Read the model definition and answer for the solid it produces. Units are mm, in the model's axes. Face numbers are marked on the shaded views. A direction names the side the tool comes from. Coordinates: 2 decimals unless noted, no trailing zeros. Order: outer loops, then holes, each group sorted by start corner. A loop starts at its lowest first (then second) coordinate and runs counter-clockwise, first axis right, second up.
```python
from build123d import *

# Parameters (mm, degrees)
SKETCH1_R           = 17
BOSS_EXTRUDE1_DEPTH = 14
SKETCH2_R           = 12.9
CUT_EXTRUDE1_DEPTH  = 10.5
SKETCH3_R           = 11
CUT_EXTRUDE3_DEPTH  = 28.820855486


with BuildPart() as part:
    # Sketch1 → Boss-Extrude1 (new body)
    with BuildSketch(Plane.XY):
        Circle(SKETCH1_R)
    extrude(amount=BOSS_EXTRUDE1_DEPTH)

    # Sketch2 → Cut-Extrude1 (cut)
    with BuildSketch(Plane.XY):
        with Locations(Location((0, 0, 0), (0, 0, 180))):
            Circle(SKETCH2_R)
    extrude(amount=CUT_EXTRUDE1_DEPTH, mode=Mode.SUBTRACT)

    # Sketch3 → Cut-Extrude3 (cut, through all)
    with BuildSketch(Plane.XY):
        Circle(SKETCH3_R)
    extrude(amount=CUT_EXTRUDE3_DEPTH, mode=Mode.SUBTRACT)


solid = part.part
```
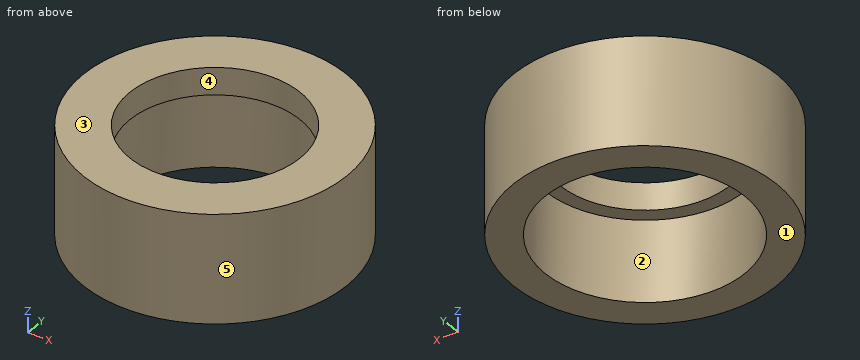
1) Straight lines are drawn through the part: line 1 (Y direction, x = 0, z = 5); line 2 (Y direction, x = 0, z = 11.4); line 3 (Z direction, x = -10.5, y = 6.5). For each, find the intervals that lie inside material, in ascending order.
A:
line 1: y = -17 to -12.9, 12.9 to 17
line 2: y = -17 to -11, 11 to 17
line 3: z = 10.5 to 14
2) A cutting plane is placed at B-B, the plane x = -4. Determine the outline of the cut face in (y, z).
A:
outline: (-16.52, 0) - (-12.26, 0) - (-12.26, 10.5) - (-10.25, 10.5) - (-10.25, 14) - (-16.52, 14) - close; (10.25, 10.5) - (12.26, 10.5) - (12.26, 0) - (16.52, 0) - (16.52, 14) - (10.25, 14) - close
3) Flat-ended cylindrical pins translate along their axes: pin 1 Ø1 at (y, z) = (-13, 9) entering from +X; pin 2 Ø15.5 at (x, y) = (0, 0) entering from -Z; pin 3 Ø2 at (y, z) = (-4, 5.5) entering from -X; pin 4 Ø3 at (y, z) = (-1, 4) entering from +X. Find the tip coordinate at first contact, or state that the pin passes through.
A:
pin 1: stops at x = 11.52
pin 2: passes through
pin 3: stops at x = -16.73
pin 4: stops at x = 17
4) A cutting plane is placed at C-C, the plane z = 12.75. Determine the outline of the cut face in (x, y), and give its area (3 significant figures).
A:
outline: circle Ø34 at (0, 0); hole circle Ø22 at (0, 0)
area: 528 mm2
5) Which of the six approach directions +Z, -Z, +X, -X, +Y, -Y give full straight-line access (tool end or side, diameter ignored) to the marked faces 1 and 2?
A:
face 1: -Z, +X, -X, +Y, -Y
face 2: -Z
6) A cutting plane is placed at A-A, the plane y = 0. Determine the outline of the cut face in (x, z).
A:
outline: (-17, 0) - (-12.9, 0) - (-12.9, 10.5) - (-11, 10.5) - (-11, 14) - (-17, 14) - close; (11, 10.5) - (12.9, 10.5) - (12.9, 0) - (17, 0) - (17, 14) - (11, 14) - close
7) A cutting plane is placed at D-D, the plane x = 13.5. Determine the outline of the cut face in (y, z), and give its area (3 significant figures).
A:
outline: (-10.33, 0) - (10.33, 0) - (10.33, 14) - (-10.33, 14) - close
area: 289 mm2
8) Determine the mould class of the marked faces 3, 4 and 5 for opening direction X: pulls with the +X half, pulls with the -X half, needs draft (parallel to the pull), parting line crosses it, or undercut.
A:
face 3: needs draft
face 4: undercut
face 5: parting line crosses it
